CAD build for the part. Positions are in the model's coordinates, mm. Face numbers are marked on the shaded views. Give positions to 0.01 mm unless a question says otherwise; leave off trailing zeros. Order: outer loops, then holes, each group sorted by start corner. A loop starts at its lowest first (then second) coordinate and runs counter-clockwise, first axis right, second up.
Item 1: Flat gauge pins, fed straight in: P1, Ø3.5, axis at y = 19, z = 22, coming from the -X side; P2, Ø8, axis at y = -1, z = 17, coming from the -X side; P3, Ø6.5, axis at y = 19, z = 4, coming from the -X side; P4, Ø5, axis at x = -9, y = -14.5, coming from the +Z side. Where does each tip first touch, or does it go through?
Item 2: Band-saw the part on C-C on z = 9. Give the cut face in (x, y).
Item 3: Wall check: L1, parallel to Y at x = 10.5, z = 22; L2, parallel to Z at x = 11.25, y = 19; L3, parallel to Z at x = 6, y = 19. Give the ranges that are in metal, low to high.
Item 4: Band-saw the part on D-D on y = -12. Give the cut face in (x, z).
Item 5: Band-saw the part on A-A on x = 0. Give the cut face in (y, z).
Item 6: Band-saw the part on B-B on x = 6. Give the cut face in (y, z), plus the area to 3 significant figures.
Item 7: Two-plate mould, pull along Z, no slides. Class the marked faces 1, 2 and 3: released by +Z, released by -Z, zero draft, split by the parting line, or undercut.
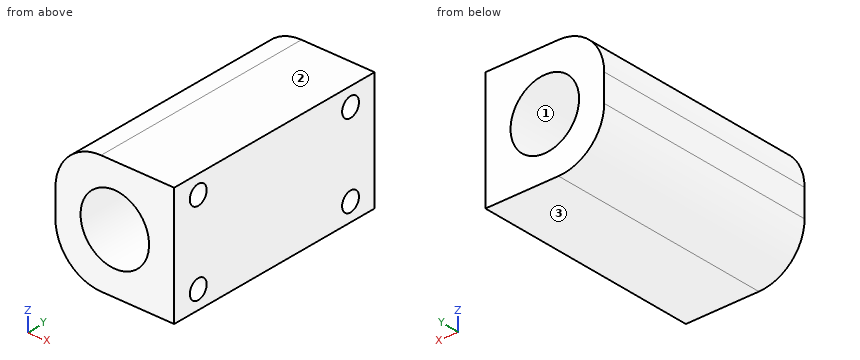
```python
from build123d import *

# Parameters (mm, degrees)
SKIZZE1_W                       = 26
SKIZZE1_H                       = 50
AUFSATZ_LINEAR_AUSTRAGEN1_DEPTH = 26
VERRUNDUNG1_R                   = 10
SKIZZE2_R                       = 7.5
SCHNITT_LINEAR_AUSTRAGEN1_DEPTH = 58.835974964
M5_GEWINDEBOHRUNG1_D            = 4.2
M5_GEWINDEBOHRUNG1_DEPTH        = 9
M5_GEWINDEBOHRUNG1_TIP          = 1.2618073


with BuildPart() as part:
    # Skizze1 → Aufsatz-Linear austragen1 (new body)
    with BuildSketch(Plane.XY):
        Rectangle(SKIZZE1_W, SKIZZE1_H)
    extrude(amount=AUFSATZ_LINEAR_AUSTRAGEN1_DEPTH)

    # Verrundung1
    verrundung1_edges = [part.edges().sort_by_distance(p)[0] for p in [
        (-13, 0, 26),
        (-13, 0, 0),
    ]]
    fillet(verrundung1_edges, radius=VERRUNDUNG1_R)

    # Skizze2 → Schnitt-Linear austragen1 (cut, through all)
    with BuildSketch(Plane(origin=(0, 25, 0), x_dir=(1, 0, 0), z_dir=(0, 1, 0))):
        with Locations(Location((0, -13, 0), (0, 0, 180))):
            Circle(SKIZZE2_R)
    extrude(amount=-SCHNITT_LINEAR_AUSTRAGEN1_DEPTH, mode=Mode.SUBTRACT)

    # M5 Gewindebohrung1
    with Locations(Plane(origin=(13, 0, 0), x_dir=(0, 0, -1), z_dir=(1, 0, 0))):
        with Locations((-22, 19), (-4, 19), (-22, -19), (-4, -19)):
            Hole(M5_GEWINDEBOHRUNG1_D / 2, depth=M5_GEWINDEBOHRUNG1_DEPTH)
            with Locations((0, 0, -(M5_GEWINDEBOHRUNG1_DEPTH + M5_GEWINDEBOHRUNG1_TIP / 2))):  # 118° drill point
                Cone(0, M5_GEWINDEBOHRUNG1_D / 2, M5_GEWINDEBOHRUNG1_TIP, mode=Mode.SUBTRACT)


solid = part.part
```
The answers:
1. P1: stops at x = -12.05
1. P2: stops at x = -13
1. P3: stops at x = -12.61
1. P4: stops at z = 25.37
2. outline: (-12.95, -25) - (-6.34, -25) - (-6.34, 25) - (-12.95, 25) - close; (6.34, -25) - (13, -25) - (13, 25) - (6.34, 25) - close
3. L1: y = -25 to -21.1, -16.9 to 16.9, 21.1 to 25
3. L2: z = 0 to 1.9, 6.1 to 19.9, 24.1 to 26
3. L3: z = 0 to 1.9, 6.1 to 8.5, 17.5 to 19.9, 24.1 to 26
4. outline: (-13, 10) arc R10 ccw to (-3, 0) - (13, 0) - (13, 26) - (-3, 26) arc R10 ccw to (-13, 16) - close; hole circle Ø15 at (0, 13)
5. outline: (-25, 0) - (25, 0) - (25, 5.5) - (-25, 5.5) - close; (-25, 20.5) - (25, 20.5) - (25, 26) - (-25, 26) - close
6. outline: (-25, 0) - (25, 0) - (25, 8.5) - (-25, 8.5) - close; (-25, 17.5) - (25, 17.5) - (25, 26) - (-25, 26) - close; hole circle Ø4.2 at (-19, 4); hole circle Ø4.2 at (-19, 22); hole circle Ø4.2 at (19, 4); hole circle Ø4.2 at (19, 22)
6. area: 795 mm2
7. face 1: undercut
7. face 2: released by +Z
7. face 3: released by -Z
